The listing builds one solid part. Answer for the finished solid, in the listing's coordinates (mm). Coordinates: 2 decimals unless noted, no trailing zeros. Order: outer loops, then holes, each group sorted by start corner. A loop starts at its lowest first (then second) coordinate and runs counter-clockwise, first axis right, second up. Notation, with made-up numbers: (32.5, 25) - (54.5, 25) arc R24 cw to (54.5, 38) - close; hole circle Ø5 at (7, 55.5). An arc over 180 degrees is marked (long way). Use a Markdown table: item, result. Add a question column.
Item 1: The part is cut by section C-C, the plane z = 5.25. Give the vertices of the cut face in (x, y), then the cut area to 3 significant figures.
Item 2: Find the intervals of material crossed by line 1 along Y through (x, z) = (0, 1.3); line 2 along Y through (x, z) = (9, 3.5), in increasing order.
Item 3: Flat-ended cylindrical pins translate along their axes: P1, Ø2, axis at y = -8.5, z = 3.5, coming from the -X side; P2, Ø3, axis at x = -26.5, z = 1.5, coming from the -Y side; P3, Ø5, axis at x = 28.5, y = -30, coming from the +Z side. Find the tip coordinate at first contact, or state that the pin passes through.
Item 4: The mould has two halves that part along Y. Classify faces 1 (the conical face through (-18.77, -29.43, 6.85)), 2 (the flat face through (-20, 20, 0)), 3 (the cylindrical face through (-44.83, -14.12, 1.97)): released by +Y, released by -Y, zero draft, split by the parting line, or undercut.
from build123d import *


with BuildPart() as f1:
    # F0 (on Front) → F1 (revolve)
    with BuildSketch(Plane.XZ):
        with BuildLine():
            Line((-47, 0), (-25, 0))
            Line((-25, 0), (-25, 3.982928))
            Line((-25, 3.982928), (-25.021957, 4))
            Line((-25.021957, 4), (-25, 4))
            Line((-25, 4), (-26.90827, 6.454344))
            ThreePointArc((-26.90827, 6.454344), (-28.136784, 7.153221), (-29.499656, 6.778711))
            Line((-29.499656, 6.778711), (-33.024692, 4.037971))
            Line((-33.024692, 4.037971), (-33.054214, 4))
            Line((-33.054214, 4), (-33.073528, 4))
            Line((-33.073528, 4), (-34.178294, 7.034632))
            ThreePointArc((-34.178294, 7.034632), (-34.503445, 7.264412), (-34.832563, 7.040351))
            Line((-34.832563, 7.040351), (-36, 4))
            Line((-36, 4), (-37.167437, 7.040351))
            ThreePointArc((-37.167437, 7.040351), (-37.496555, 7.264412), (-37.821706, 7.034632))
            Line((-37.821706, 7.034632), (-38.926472, 4))
            Line((-38.926472, 4), (-42.500344, 6.778711))
            ThreePointArc((-42.500344, 6.778711), (-43.863216, 7.153221), (-45.09173, 6.454344))
            Line((-45.09173, 6.454344), (-47, 4))
            Line((-47, 4), (-47, 0))
        make_face()
        Polygon((-25.021957, 4), (-25, 3.982928), (-25, 4), align=None)
        Polygon((-33.054214, 4), (-33.024692, 4.037971), (-33.073528, 4), align=None)
    revolve(axis=Axis((0, 0, 2), (0, 0, 1)))


solid = f1.part
Solution:
| question | item | result |
|---|---|---|
| 1 | outline | circle Ø92.06 at (0, 0); circle Ø76.94 at (0, 0); circle Ø71.04 at (0, 0); circle Ø62.93 at (0, 0); hole circle Ø81.07 at (0, 0); hole circle Ø72.96 at (0, 0); hole circle Ø67.06 at (0, 0); hole circle Ø51.94 at (0, 0) |
| 1 | area | 3,390 mm2 |
| 2 | line 1 | y = -47 to -25, 25 to 47 |
| 2 | line 2 | y = -46.13 to -23.32, 23.32 to 46.13 |
| 3 | P1 | stops at x = -46.4 |
| 3 | P2 | stops at y = -39.8 |
| 3 | P3 | stops at z = 7.17 |
| 4 | face 1 | undercut |
| 4 | face 2 | zero draft |
| 4 | face 3 | split by the parting line |
